from build123d import *

# Parameters (mm, degrees)
PAD_DEPTH       = 4.45
SKETCH001_W     = 18
SKETCH001_H     = 70
POCKET_DEPTH    = 3.45
SKETCH002_R     = 3.075
PAD001_DEPTH    = 6
POCKET001_DEPTH = 6
SKETCH004_W     = 21.675
SKETCH004_H     = 8.5
POCKET002_DEPTH = 4.1


with BuildPart() as part:
    # Sketch → Pad (new body)
    with BuildSketch(Plane.XY):
        with BuildLine():
            Line((-30.675, 44.765), (-30.675, -44.765))
            ThreePointArc((-30.675, -44.765), (-29.210534, -48.300534), (-25.675, -49.765))
            Line((-25.675, -49.765), (25.675, -49.765))
            ThreePointArc((25.675, -49.765), (29.210534, -48.300534), (30.675, -44.765))
            Line((30.675, -44.765), (30.675, 44.765))
            ThreePointArc((30.675, 44.765), (29.210534, 48.300534), (25.675, 49.765))
            Line((25.675, 49.765), (-25.675, 49.765))
            ThreePointArc((-25.675, 49.765), (-29.210534, 48.300534), (-30.675, 44.765))
        make_face()
    extrude(amount=PAD_DEPTH)

    # Sketch001 (on Face10 of Pad) → Pocket (cut)
    with BuildSketch(Plane.XY.offset(4.45)):
        with Locations((0, 14.765)):
            Rectangle(SKETCH001_W, SKETCH001_H)
    extrude(amount=-POCKET_DEPTH, mode=Mode.SUBTRACT)

    # Sketch002 (on Face5 of Pocket) → Pad001 (join)
    with BuildSketch(Plane.XY.offset(4.45)):
        with Locations((-20.175, 38.265)):
            Circle(SKETCH002_R)
        with Locations((20.175, 38.265)):
            Circle(SKETCH002_R)
        with Locations((-20.175, -42.265)):
            Circle(SKETCH002_R)
        with Locations((20.175, -42.265)):
            Circle(SKETCH002_R)
    extrude(amount=PAD001_DEPTH)

    # Sketch003 (on Face21 of Pad001) → Pocket001 (cut)
    with BuildSketch(Plane.XY.offset(10.45)):
        Polygon((-21.058883, 42.348883), (-21.058883, 39.148883), (-24.258883, 39.148883), (-24.258883, 37.381117), (-21.058883, 37.381117), (-21.058883, 34.181117), (-19.291117, 34.181117), (-19.291117, 37.381117), (-16.091117, 37.381117), (-16.091117, 39.148883), (-19.291117, 39.148883), (-19.291117, 42.348883), align=None)
        Polygon((21.058883, 42.348883), (21.058883, 39.148883), (24.258883, 39.148883), (24.258883, 37.381117), (21.058883, 37.381117), (21.058883, 34.181117), (19.291117, 34.181117), (19.291117, 37.381117), (16.091117, 37.381117), (16.091117, 39.148883), (19.291117, 39.148883), (19.291117, 42.348883), align=None)
        Polygon((-21.058883, -46.508146), (-21.058883, -43.148883), (-24.418146, -43.148883), (-24.418146, -41.381117), (-21.058883, -41.381117), (-21.058883, -38.021854), (-19.291117, -38.021854), (-19.291117, -41.381117), (-15.931854, -41.381117), (-15.931854, -43.148883), (-19.291117, -43.148883), (-19.291117, -46.508146), align=None)
        Polygon((21.058883, -47.109884), (21.058883, -43.148883), (25.019884, -43.148883), (25.019884, -41.381117), (21.058883, -41.381117), (21.058883, -37.420116), (19.291117, -37.420116), (19.291117, -41.381117), (15.330116, -41.381117), (15.330116, -43.148883), (19.291117, -43.148883), (19.291117, -47.109884), align=None)
    extrude(amount=-POCKET001_DEPTH, mode=Mode.SUBTRACT)

    # Sketch004 (on Face14 of Pocket001) → Pocket002 (cut)
    with BuildSketch(Plane.XY.offset(4.45)):
        with Locations((19.8375, 19.015)):
            Rectangle(SKETCH004_W, SKETCH004_H)
    extrude(amount=-POCKET002_DEPTH, mode=Mode.SUBTRACT)


solid = part.part
Here's how the part is built. I have some questions about the finished solid (model axes, mm). A direction names the side the tool comes from. Coordinates: 2 decimals unless noted, no trailing zeros. Write each loop counter-clockwise with the first axis right and the second up, starting at its lowest first coordinate (ties: lowest second). Pieces come first, ordered by that corner, then holes.
Item 1: I want a section at C-C on z = 8.25. Count the separate pieces of the cut face and the enclosed holes in it, and give its area (3 significant figures).
Item 2: If we mould it in two halves opening along Y, with no side actions, what happens to faces 1 (the cylindrical face through (-22.334, 40.454, 7.408)), 2 (the flat face through (20, 23.265, 2)), 3 (the flat face through (19.291, -44, 7))? For each: +Y half, -Y half, draft (parallel to the pull), parting line (faces both ways), or undercut.
Item 3: I want a section at D-D on x = 27.5. Write out the boundary of the cut face in (y, z) (3 decimals).
Item 4: Will these pins go through, and if not, where does the flat tip stop? pin 1 (0.6 mm diameter, centred on y = -44.5, z = 9, fed in from +X); pin 2 (2 mm diameter, centred on x = -11.5, y = -28, fed in from +Z); pin 3 (0.6 mm diameter, centred on y = -44.5, z = 8, fed in from -X).
Item 5: On a 3-axis mill with a long thin cutter (end or side, diameter ignored), from which of +Z, -Z, +X, -X, +Y, -Y can I reach the whole of each face in a straight line? I mean faces 4 (the flat face through (18, -43.149, 7)), 5 (the cylindrical face through (22.364, 40.424, 7.408)), 6 (the flat face through (-19.291, 40, 7)). Say none if no direction works.
Item 6: I want a section at B-B on y = 3.5. Write out the boundary of the cut face in (x, z) (3 decimals).
Item 7: If I drill on line 1 (X direction, y = -40.5, z = 7.25); line 2 (Y direction, x = 23, z = 6.5); line 3 (X direction, y = 35.5, z = 1.5) (3 decimals), over which ranges is the centre line in solid material (lowest first)?
Item 8: I want a section at A-A on z = 2.25. Write out the boundary of the cut face in (x, y) (3 decimals), and give its area (3 significant figures).
Findings below:
1. separate pieces: 16
1. enclosed holes: 0
1. area: 45.6 mm2
2. face 1: +Y half
2. face 2: undercut
2. face 3: draft
3. outline: (-49.42, 0) - (49.42, 0) - (49.42, 4.45) - (23.265, 4.45) - (23.265, 0.35) - (14.765, 0.35) - (14.765, 4.45) - (-49.42, 4.45) - close
4. pin 1: stops at x = 22.56
4. pin 2: stops at z = 4.45
4. pin 3: stops at x = -22.56
5. face 4: +Z, +X, -X
5. face 5: +Z, +X, +Y
5. face 6: +Z, +Y, -Y
6. outline: (-30.675, 0) - (30.675, 0) - (30.675, 4.45) - (9, 4.45) - (9, 1) - (-9, 1) - (-9, 4.45) - (-30.675, 4.45) - close
7. line 1: x = -22.69 to -21.06, -19.29 to -17.66, 17.66 to 19.29, 21.06 to 22.69
7. line 2: y = -43.48 to -43.15, -41.38 to -41.05, 37.05 to 37.38, 39.15 to 39.48
7. line 3: x = -30.675 to -9, 9 to 30.675
8. outline: (-30.675, -44.765) arc R5 ccw to (-25.675, -49.765) - (25.675, -49.765) arc R5 ccw to (30.675, -44.765) - (30.675, 14.765) - (9, 14.765) - (9, -20.235) - (-9, -20.235) - (-9, 49.765) - (-25.675, 49.765) arc R5 ccw to (-30.675, 44.765) - close; (9, 23.265) - (30.675, 23.265) - (30.675, 44.765) arc R5 ccw to (25.675, 49.765) - (9, 49.765) - close
8. area: 4,640 mm2
